CAD build for the part. Positions are in the model's coordinates, mm. A direction names the side the tool comes from. Round coordinates to 2 decimals unless told otherwise and drop trailing zeros. Write each loop counter-clockwise with the first axis right and the second up, starting at its lowest first coordinate (ties: lowest second). Pieces come first, ordered by that corner, then holes. Notation, with made-up numbers: (-34, -38) -> (-16, -38) arc R15 cw to (-16, -10) -> close; hole circle Ø6 at (-24.75, 71). An arc over 180 degrees is marked (long way). Answer in a Markdown table with one row per item. Add a question column.
```python
from build123d import *

# Parameters (mm, degrees)
SKETCH010_W           = 350
SKETCH010_H           = 330
PAD002_DEPTH          = 5
PAD003_DEPTH          = 5
SKETCH012_R           = 1.5
POCKET004_DEPTH       = 5
POLARPATTERN_COUNT    = 2
POLARPATTERN001_COUNT = 2
FILLET004_R           = 1
SKETCH013_R           = 117.5
POCKET005_DEPTH       = 10


with BuildPart() as part:
    # Sketch010 → Pad002 (new body)
    with BuildSketch(Plane.XY):
        Rectangle(SKETCH010_W, SKETCH010_H)
    extrude(amount=PAD002_DEPTH)

    # Sketch011 → Pad003 (join)
    with BuildSketch(Plane.YZ.offset(175)):
        with BuildLine():
            Line((-160, 0), (-160, 15))
            ThreePointArc((-140, 15), (-150, 25), (-160, 15))
            Line((-140, 15), (-140, 0))
            Line((-140, 0), (-160, 0))
        make_face()
    pad003 = extrude(amount=-PAD003_DEPTH)

    # Sketch012 → Pocket004 (cut)
    with BuildSketch(Plane.YZ.offset(175)):
        with Locations((-150, 15)):
            Circle(SKETCH012_R)
    pocket004 = extrude(amount=-POCKET004_DEPTH, mode=Mode.SUBTRACT)

    # Mirrored: Pad003 across Sketch011 V_Axis
    add(pad003.mirror(Plane(origin=(175, 0, 0), x_dir=(1, 0, 0), z_dir=(0, 1, 0))))

    # Mirrored001: Pocket004 across Sketch012 V_Axis
    add(pocket004.mirror(Plane(origin=(175, 0, 0), x_dir=(1, 0, 0), z_dir=(0, 1, 0))), mode=Mode.SUBTRACT)

    # Mirrored002: Pad003 across YZ
    add(pad003.mirror(Plane.YZ))

    # Mirrored003: Pocket004 across YZ
    add(pocket004.mirror(Plane.YZ), mode=Mode.SUBTRACT)

    # PolarPattern: Pad003 ×2 about axis
    polarpattern_axis = Axis((0, 0, 0), (0, 0, 1))
    for i in range(1, POLARPATTERN_COUNT):
        add(pad003.rotate(polarpattern_axis, i * 360 / POLARPATTERN_COUNT))

    # PolarPattern001: Pocket004 ×2 about axis
    polarpattern001_axis = Axis((0, 0, 0), (0, 0, 1))
    for i in range(1, POLARPATTERN001_COUNT):
        add(pocket004.rotate(polarpattern001_axis, i * 360 / POLARPATTERN001_COUNT), mode=Mode.SUBTRACT)

    # Fillet004
    fillet004_edges = [part.edges().sort_by_distance(p)[0] for p in [
        (0, 165, 0),
        (175, 0, 0),
        (0, -165, 0),
        (-175, 0, 0),
    ]]
    fillet(fillet004_edges, radius=FILLET004_R)

    # Sketch013 → Pocket005 (cut)
    with BuildSketch(Plane.XY):
        Circle(SKETCH013_R)
    extrude(amount=POCKET005_DEPTH, mode=Mode.SUBTRACT)


solid = part.part
```
Item 1: Pin check, flat tips, straight feed: pin 1 (2 mm diameter, centred on x = 17.5, y = 126, fed in from +Z); pin 2 (1.5 mm diameter, centred on x = 173.5, z = 8.5, fed in from +Y); pin 3 (4 mm diameter, centred on x = -171.5, z = 11.5, fed in from -Y). Stop position of each tip, or through.
Item 2: Saw through at B-B on x = 0. Give the cut face in (y, z).
Item 3: Tool access for faces 1 (the flat face through (-170, -150, 13)), 2 (the cylindrical face through (173, -150, 25)): list every direction of +Z, -Z, +X, -X, +Y, -Y with a clear straight run to the whole face (end or side of a thin tool).
Item 4: Drill centre lines: probe 1 along Y at (x, z) = (0, 1.1); probe 2 along Z at (x, y) = (171, -150); probe 3 along X at (y, z) = (0, 3). Where is each one in solid material? Low to high.
Item 5: Saw through at C-C on x = 140. Give the cut face in (y, z), then the cut area to 3 significant figures.
Item 6: Two-plate mould, pull along X, no slides. Class faces 3 (the flat face through (170, -150, 13)), 4 (the flat face through (175, -2.3, 4.8)), 5 (the flat face through (-41, -112, 0)): +X half, -X half, draft (parallel to the pull), parting line (faces both ways), or undercut.
Item 7: Saw through at A-A on y = 0. Give the cut face in (x, z), then the cut area to 3 significant figures.
Recorded:
| question | item | result |
|---|---|---|
| 1 | pin 1 | z = 5 |
| 1 | pin 2 | y = 160 |
| 1 | pin 3 | y = -160 |
| 2 | outline | (-165, 1) arc R1 ccw to (-164, 0) -> (-117.5, 0) -> (-117.5, 5) -> (-165, 5) -> close; (117.5, 0) -> (164, 0) arc R1 ccw to (165, 1) -> (165, 5) -> (117.5, 5) -> close |
| 3 | face 1 | +Z, +Y, -Y |
| 3 | face 2 | +Z, +X, -X |
| 4 | probe 1 | -165 to -117.5, 117.5 to 165 |
| 4 | probe 2 | 0 to 13.5, 16.5 to 25 |
| 4 | probe 3 | -175 to -117.5, 117.5 to 175 |
| 5 | outline | (-165, 1) arc R1 ccw to (-164, 0) -> (164, 0) arc R1 ccw to (165, 1) -> (165, 5) -> (-165, 5) -> close |
| 5 | area | 1,650 mm2 |
| 6 | face 3 | undercut |
| 6 | face 4 | +X half |
| 6 | face 5 | draft |
| 7 | outline | (-175, 1) arc R1 ccw to (-174, 0) -> (-117.5, 0) -> (-117.5, 5) -> (-175, 5) -> close; (117.5, 0) -> (174, 0) arc R1 ccw to (175, 1) -> (175, 5) -> (117.5, 5) -> close |
| 7 | area | 575 mm2 |
